from build123d import *

# Parameters (mm, degrees)
SKETCH1_R           = 1.1
BOSS_EXTRUDE1_DEPTH = 3.175
CHAMFER1_SIZE       = 15


with BuildPart() as part:
    # Sketch1 → Boss-Extrude1 (new body)
    # profile 1 of 2: a face of its own
    with BuildSketch(Plane.XY):
        Polygon((10.8, 21.8), (10.8, 34), (3.175, 34), (3.175, 26), (0, 26), (0, 19.9), (3.175, 19.9), (3.175, 17), (40, 17), (40, 34), (34, 34), (34, 21.8), align=None)
        with Locations((8.65, 27.9)):
            Circle(SKETCH1_R, mode=Mode.SUBTRACT)
        with Locations((36.15, 27.9)):
            Circle(SKETCH1_R, mode=Mode.SUBTRACT)
    # profile 2 of 2: a face of its own
    with BuildSketch(Plane.XY):
        Polygon((40, 0), (40, 17), (3.175, 17), (3.175, 15), (8.5, 15), (8.5, 16.625), (12, 16.625), (12, 15), (20, 15), (20, 11), (12, 11), (12, 9.375), (8.5, 9.375), (8.5, 11), (3.175, 11), (3.175, 6.1), (0, 6.1), (0, 0), align=None)
    extrude(amount=BOSS_EXTRUDE1_DEPTH)

    # Chamfer1
    chamfer1_edges = [part.edges().sort_by_distance(p)[0] for p in [
        (40, 0, 1.5875),
    ]]
    chamfer(chamfer1_edges, length=CHAMFER1_SIZE)


solid = part.part
Design review of the part built by this model. Coordinates are the model's own, in mm. A direction names the side the tool comes from. Coordinates: 2 decimals unless noted, no trailing zeros. Write each loop counter-clockwise with the first axis right and the second up, starting at its lowest first coordinate (ties: lowest second). Pieces come first, ordered by that corner, then holes. Notation, with made-up numbers: (31, -12.75) - (62, -12.75) arc R12 cw to (62, -5.75) - close; hole circle Ø7 at (-11, 72). An arc over 180 degrees is marked (long way). Use one line per item in the form item = value.
Q1. Consider section C-C (y = 10). Write out the cut boundary in (x, z) (3 decimals).
Taken from the geometry:
outline = (3.175, 0) - (8.5, 0) - (8.5, 3.175) - (3.175, 3.175) - close; (12, 0) - (35, 0) - (35, 3.175) - (12, 3.175) - close
Q2. The part is to be moulded in two halves that separate along Y. For faces 6 (the flat face through (12, 0, 2)), 7 (the flat face through (20, 17, 0)), 8 (the flat face through (8.5, 16, 2)), say which applies: +Y half, -Y half, draft (parallel to the pull), parting line (faces both ways), or undercut.
Taken from the geometry:
face_6 = -Y half
face_7 = draft
face_8 = undercut
Q3. Consider section A-A (y = 27.9). Write out the cut boundary in (x, z) (3 decimals), plus the area to 3 significant figures.
Taken from the geometry:
outline = (3.175, 0) - (7.55, 0) - (7.55, 3.175) - (3.175, 3.175) - close; (9.75, 0) - (10.8, 0) - (10.8, 3.175) - (9.75, 3.175) - close; (34, 0) - (35.05, 0) - (35.05, 3.175) - (34, 3.175) - close; (37.25, 0) - (40, 0) - (40, 3.175) - (37.25, 3.175) - close
area = 29.3 mm^2
Q4. Machinability: for faces 1 (the flat face through (3.175, 30, 2)), 2 (the flat face through (16, 15, 2)), 3 (the flat face through (12, 10, 2)), 4 (the flat face through (34, 28, 2)), 5 (the flat face through (0, 23, 2)), which of the approach directions +Z, -Z, +X, -X, +Y, -Y give a long, thin tool a straight path to every point of the face, cutting with its end or side? Answer none if there is none.
Taken from the geometry:
face_1 = +Z, -Z, -X, +Y
face_2 = +Z, -Z, -X
face_3 = +Z, -Z
face_4 = +Z, -Z, +Y
face_5 = +Z, -Z, -X, +Y, -Y
Q5. Consider section B-B (x = 36.15). Write out the cut boundary in (y, z) (3 decimals), plus the area to 3 significant figures.
Taken from the geometry:
outline = (11.15, 0) - (26.8, 0) - (26.8, 3.175) - (11.15, 3.175) - close; (29, 0) - (34, 0) - (34, 3.175) - (29, 3.175) - close
area = 65.6 mm^2
Q6. Insertion check: pin 1 Ø1 at (y, z) = (13, 2) entering from -X; pin 2 Ø1.3 at (y, z) = (10, 2.5) entering from +X; pin 3 Ø1 at (y, z) = (8.5, 1) entering from -X (3 decimals); pin 4 Ø1.5 at (y, z) = (20, 0.5) entering from -X. Each pin has a flat end and moves straight along its axis. Give the tip position at first contact, or say it passes through.
Taken from the geometry:
pin_1 = 20
pin_2 = 35.65
pin_3 = 3.175
pin_4 = 0
Q7. For probe 1 along Y at (x, z) = (8.65, 1.55) (3 decimals); probe 2 along Y at (x, z) = (15, 1.85); probe 3 along X at (y, z) = (24.5, 1.7), list the stretches that pass through material, from the lowest coordinate up.
Taken from the geometry:
probe_1 = 0 to 9.375, 16.625 to 26.8, 29 to 34
probe_2 = 0 to 11, 15 to 21.8
probe_3 = 0 to 10.8, 34 to 40
Q8. Consider section D-D (z = 1.6). Count the separate pieces of the cut face and the enclosed holes in it, plus the area to 3 significant figures.
Taken from the geometry:
separate_pieces = 1
enclosed_holes = 2
area = 809 mm^2
